Input: part model. Units: mm. Frame: model coordinates. A direction names the side the tool comes from. Give positions to 0.01 mm unless a question says otherwise; leave off trailing zeros. Write each loop counter-clockwise with the first axis right and the second up, starting at its lowest first coordinate (ties: lowest second). Pieces come first, ordered by that corner, then holes. Notation, with made-up numbers: (-13.5, 16.25) - (30.5, 16.25) arc R18 cw to (30.5, 28.25) - close; hole circle Ø9 at (-6, -8). An arc over 180 degrees is marked (long way). Answer as CSV lines item,"result". Start each with the question number.
from build123d import *

# Parameters (mm, degrees)
SKETCH1_R               = 1.6
BOSS_EXTRUDE1_DEPTH     = 2
BOSS_EXTRUDE2_START     = -8
SKETCH1_3_R             = 1.6
BOSS_EXTRUDE2_DEPTH     = 8
SKETCH2_R               = 5
CUT_EXTRUDE1_DEPTH      = 5
SKETCH7_R               = 1.6
BOSS_EXTRUDE5_DEPTH     = 2
BOSS_EXTRUDE6_START     = -8
BOSS_EXTRUDE6_OUTLINE_R = 1.6
BOSS_EXTRUDE6_DEPTH     = 8
CUT_EXTRUDE4_START      = 5
SKETCH8_R               = 5
CUT_EXTRUDE4_DEPTH      = 5
SKETCH10_R              = 3.5
SKETCH10_R_2            = 1.6
CUT_EXTRUDE5_DEPTH      = 1
FILLET2_R               = 0.5
FILLET3_R               = 0.3
CUT_EXTRUDE6_START      = -1
SKETCH11_R              = 3.5
SKETCH11_R_2            = 1.6
CUT_EXTRUDE6_DEPTH      = 1
FILLET4_R               = 0.3


# Read off the part's stored shape, not the designer's step: Boss-Extrude6
with BuildPart() as part:
    # Sketch1 → Boss-Extrude1 (new body)
    with BuildSketch(Plane.XY):
        with BuildLine():
            Line((13.181503179, 9.65917228), (9.685706637, 13.234001861))
            Line((9.685706637, 13.234001861), (1.09631205, 4.834503308))
            ThreePointArc((1.09631205, 4.834503308), (-3.826512492, -3.476156637), (4.592108592, 1.259673726))
            Line((4.592108592, 1.259673726), (13.181503179, 9.65917228))
        make_face()
        with Locations((-0.251682911, 0.019639905)):
            Circle(SKETCH1_R, mode=Mode.SUBTRACT)
    extrude(amount=BOSS_EXTRUDE1_DEPTH)

    # Sketch1<3> → Boss-Extrude2 (add)
    with BuildSketch(Plane.XY.offset(BOSS_EXTRUDE2_START)):
        with BuildLine():
            Line((13.181503179, 9.65917228), (9.685706637, 13.234001861))
            Line((9.685706637, 13.234001861), (1.09631205, 4.834503308))
            ThreePointArc((1.09631205, 4.834503308), (-3.826512492, -3.476156637), (4.592108592, 1.259673726))
            Line((4.592108592, 1.259673726), (13.181503179, 9.65917228))
        make_face()
        with Locations(Location((-0.251682911, 0.019639905, 0), (0, 0, 180))):
            Circle(SKETCH1_3_R, mode=Mode.SUBTRACT)
    extrude(amount=BOSS_EXTRUDE2_DEPTH)

    # Sketch2 → Cut-Extrude1 (cut)
    with BuildSketch(Plane(origin=(0, 0, -6), x_dir=(-1, 0, 0), z_dir=(0, 0, -1))):
        with Locations((0.251682911, 0.019639905)):
            Circle(SKETCH2_R)
    extrude(amount=-CUT_EXTRUDE1_DEPTH, mode=Mode.SUBTRACT)

    # Sketch7 → Boss-Extrude5 (add)
    with BuildSketch(Plane(origin=(-1.880744352, 1.923264258, 0), x_dir=(0.7149659162500773, 0.6991593084560109, 0), z_dir=(-0.6991593084560109, 0.7149659162500773, 0))):
        with BuildLine():
            Line((16.17762571, 8), (10.170769724, 8))
            Line((10.170769724, 8), (10.170769724, -2))
            Line((10.170769724, -2), (16.17762571, -2))
            ThreePointArc((16.17762571, -2), (21.17762571, 3), (16.17762571, 8))
        make_face()
        with Locations(Location((16.17762571, 3, 0), (0, 0, 270))):
            Circle(SKETCH7_R, mode=Mode.SUBTRACT)
    extrude(amount=BOSS_EXTRUDE5_DEPTH)

    # Boss-Extrude6 outline → Boss-Extrude6 (add)
    with BuildSketch(Plane(origin=(-1.880744352, 1.923264258, 0), x_dir=(0.7149659162500773, 0.6991593084560109, 0), z_dir=(-0.6991593084560109, 0.7149659162500773, 0)).offset(BOSS_EXTRUDE6_START)):
        with BuildLine():
            Line((10.170769724, 8), (10.170769724, -2))
            Line((10.170769724, -2), (16.17762571, -2))
            ThreePointArc((16.17762571, -2), (21.17762571, 3), (16.17762571, 8))
            Line((16.17762571, 8), (10.170769724, 8))
        make_face()
        with Locations((16.17762571, 3)):
            Circle(BOSS_EXTRUDE6_OUTLINE_R, mode=Mode.SUBTRACT)
    extrude(amount=BOSS_EXTRUDE6_DEPTH)

    # Sketch8 → Cut-Extrude4 (cut)
    with BuildSketch(Plane(origin=(-1.880744352, 1.923264258, 0), x_dir=(0.7149659162500772, 0.699159308456011, 0), z_dir=(0.699159308456011, -0.7149659162500772, 0)).offset(CUT_EXTRUDE4_START)):
        with Locations((16.17762571, -3)):
            Circle(SKETCH8_R)
    extrude(amount=-CUT_EXTRUDE4_DEPTH, mode=Mode.SUBTRACT)

    # Sketch10 → Cut-Extrude5 (cut)
    with BuildSketch(Plane(origin=(3.712530116, -3.796463072, 0), x_dir=(0.7149659162500772, 0.699159308456011, 0), z_dir=(0.699159308456011, -0.7149659162500772, 0))):
        with Locations((16.17762571, -3)):
            Circle(SKETCH10_R)
        with Locations((16.17762571, -3)):
            Circle(SKETCH10_R_2, mode=Mode.SUBTRACT)
    extrude(amount=-CUT_EXTRUDE5_DEPTH, mode=Mode.SUBTRACT)

    # Fillet2
    fillet2_edges = [part.edges().sort_by_distance(p)[0] for p in [
        (11.433604908, 11.446587071, 2),
        (11.433604908, 11.446587071, -8),
    ]]
    fillet(fillet2_edges, radius=FILLET2_R)

    # Fillet3
    fillet3_edges = [part.edges().sort_by_distance(p)[0] for p in [
        (4.592108592, 1.259673726, -3.5),
        (1.09631205, 4.834503308, -3.5),
    ]]
    fillet(fillet3_edges, radius=FILLET3_R)

    # Sketch11 → Cut-Extrude6 (cut)
    with BuildSketch(Plane.XY.offset(2).offset(CUT_EXTRUDE6_START)):
        with Locations((-0.251682911, 0.019639905)):
            Circle(SKETCH11_R)
        with Locations(Location((-0.251682911, 0.019639905, 0), (0, 0, 180))):
            Circle(SKETCH11_R_2, mode=Mode.SUBTRACT)
    extrude(amount=CUT_EXTRUDE6_DEPTH, mode=Mode.SUBTRACT)

    # Fillet4
    fillet4_edges = [part.edges().sort_by_distance(p)[0] for p in [
        (-3.751682911, 0.019639905, 2),
    ]]
    fillet(fillet4_edges, radius=FILLET4_R)


solid = part.part
1) Contact query for flat-ended pins moving along their axis: P1, Ø8, axis at x = 15, y = 13.5, coming from the +Z side; P2, Ø1, axis at y = -1, z = -6.5, coming from the -X side; P3, Ø6, axis at y = 10.5, z = -3, coming from the -X side. Output: stop coordinate, or through.
2) Cut plane B-B on x = 12.5. State how many separate pieces and enclosed holes the cut face has, and give its area (3 significant figures).
3) Material intervals for line 1 (Z direction, x = -4, y = 0.25); line 2 (Y direction, x = 12.5, z = -4.75); line 3 (X direction, y = 8.75, z = -1), sorted ascending. Write a range as from..to.
4) Reachability of faces 1 (the flat face through (11.224, 14.739, -2.93)), 2 (the flat face through (9.95, 4.37, -3.07)), 3 (the flat face through (1.1, 1.3, -1)) from +Z, -Z, +X, -X, +Y, -Y: full face, straight path, thin tool, end or side. Return the list, or none.
5) Pull-direction query (X, two-part tool) for faces 4 (the cylindrical face through (-0.043, -1.567, -7.014)), 5 (the cylindrical face through (17.819, 12.067, -2.89)), 6 (the flat face through (6, 5, 2)), 7 (the flat face through (6.998, 13.403, -3.07)); classes: +X half, -X half, draft (parallel to the pull), parting line (faces both ways), or undercut.
6) Cut plane A-A on z = -2. Output: boundary loops of the cut face in (x, y).
Numbers:
1,P1,"stops at z = 1.99"
1,P2,"stops at x = -5.22"
1,P3,"stops at x = 3.82"
2,separate pieces,"2"
2,enclosed holes,"1"
2,area,"44.5 mm²"
3,line 1,"z = -8..-6, -1..2"
3,line 2,"y = 4.8..6.02, 6.2..8.99, 15.99..17.06"
3,line 3,"x = 5.1..7.66, 12.25..15.11"
4,face 1,"none"
4,face 2,"+Z, -Z, -Y"
4,face 3,"-X, -Y"
5,face 4,"undercut"
5,face 5,"+X half"
5,face 6,"draft"
5,face 7,"-X half"
6,outline,"(1.45, 5.18) arc R0.3 ccw to (1.55, 4.68) arc R5 cw to (4.45, 1.72) arc R0.3 ccw to (4.94, 1.6) - (8.89, 5.46) - (10.98, 3.31) - (12.88, 5.17) - (12.18, 5.88) - (13.69, 7.36) - (12.29, 8.79) - (9.68, 6.23) - (6.18, 9.81) - (8.79, 12.36) - (7.39, 13.79) - (3.99, 10.46) - (5.39, 9.03) - close; (9.18, 15.54) - (10.58, 14.11) - (13.19, 16.66) - (11.79, 18.09) - close; (14.07, 10.53) - (15.47, 9.1) - (16.98, 10.57) - (17.68, 9.86) - (18.78, 10.94) - (16.68, 13.08) - close"
